```python
from build123d import *

# Parameters (mm, degrees)
CUT_EXTRUDE1_DEPTH      = 20.2
CUT_EXTRUDE1_DEPTH_BACK = 20.2
SKETCH3_R               = 4.05
CUT_EXTRUDE2_DEPTH      = 8.366667
SKETCH4_R               = 4.05
CUT_EXTRUDE3_DEPTH      = 8.366667


with BuildPart() as part:
    # Sketch1 → Revolve1 (revolve)
    with BuildSketch(Plane.XY):
        with BuildLine():
            Line((-1, 8.366666667), (0, 8.366666667))
            Line((0, 8.366666667), (0, 59.633333333))
            Line((0, 59.633333333), (-1, 59.633333333))
            Line((-1, 59.633333333), (-1, 67))
            ThreePointArc((-1, 67), (-1.292893219, 67.707106781), (-2, 68))
            Line((-2, 68), (-5.3, 68))
            Line((-5.3, 68), (-5.3, 57.633333333))
            ThreePointArc((-5.3, 57.633333333), (-4.557500751, 56.319940208), (-4.3, 54.833333333))
            Line((-4.3, 54.833333333), (-4.3, 51.833333333))
            Line((-4.3, 51.833333333), (-6, 51.833333333))
            Line((-6, 51.833333333), (-6, 46.833333333))
            Line((-6, 46.833333333), (-3, 46.833333333))
            Line((-3, 46.833333333), (-3, 44.333333333))
            Line((-3, 44.333333333), (-19.2, 44.333333333))
            Line((-19.2, 44.333333333), (-19.2, 41.333333333))
            Line((-19.2, 41.333333333), (-15.5, 41.333333333))
            Line((-15.5, 41.333333333), (-15.5, 23.666666667))
            Line((-15.5, 23.666666667), (-3, 23.666666667))
            Line((-3, 23.666666667), (-3, 21.166666667))
            Line((-3, 21.166666667), (-6, 21.166666667))
            Line((-6, 21.166666667), (-6, 16.166666667))
            Line((-6, 16.166666667), (-4.3, 16.166666667))
            Line((-4.3, 16.166666667), (-4.3, 13.166666667))
            ThreePointArc((-4.3, 13.166666667), (-4.557500751, 11.680059792), (-5.3, 10.366666667))
            Line((-5.3, 10.366666667), (-5.3, 0))
            Line((-5.3, 0), (-2, 0))
            ThreePointArc((-2, 0), (-1.292893219, 0.292893219), (-1, 1))
            Line((-1, 1), (-1, 8.366666667))
        make_face()
    revolve(axis=Axis((0, 0, 0), (0, 1, 0)))

    # Sketch2 → Cut-Extrude1 (cut, two sides)
    with BuildSketch(Plane.XY) as cut_extrude1_sk:
        with BuildLine():
            Line((1, 8.366666667), (0, 8.366666667))
            Line((0, 8.366666667), (0, 0))
            Line((0, 0), (2, 0))
            ThreePointArc((2, 0), (1.292893219, 0.292893219), (1, 1))
            Line((1, 1), (1, 8.366666667))
        make_face()
        with BuildLine():
            Line((-1, 8.366666667), (-1, 1))
            ThreePointArc((-1, 1), (-1.292893219, 0.292893219), (-2, 0))
            Line((-2, 0), (0, 0))
            Line((0, 0), (0, 8.366666667))
            Line((0, 8.366666667), (-1, 8.366666667))
        make_face()
        with BuildLine():
            Line((-1, 67), (-1, 59.633333333))
            Line((-1, 59.633333333), (1, 59.633333333))
            Line((1, 59.633333333), (1, 67))
            ThreePointArc((1, 67), (1.292893219, 67.707106781), (2, 68))
            Line((2, 68), (-2, 68))
            ThreePointArc((-2, 68), (-1.292893219, 67.707106781), (-1, 67))
        make_face()
    extrude(amount=CUT_EXTRUDE1_DEPTH, mode=Mode.SUBTRACT)
    extrude(cut_extrude1_sk.sketch, amount=-CUT_EXTRUDE1_DEPTH_BACK, mode=Mode.SUBTRACT)

    # Sketch3 → Cut-Extrude2 (cut)
    with BuildSketch(Plane(origin=(0, 68, 0), x_dir=(1, 0, 0), z_dir=(0, 1, 0))):
        Circle(SKETCH3_R)
    extrude(amount=-CUT_EXTRUDE2_DEPTH, mode=Mode.SUBTRACT)

    # Sketch4 → Cut-Extrude3 (cut)
    with BuildSketch(Plane.XZ):
        Circle(SKETCH4_R)
    extrude(amount=-CUT_EXTRUDE3_DEPTH, mode=Mode.SUBTRACT)


solid = part.part
```
CAD build for the part. Positions are in the model's coordinates, mm. A direction names the side the tool comes from. Coordinates: 2 decimals unless noted, no trailing zeros. Order: outer loops, then holes, each group sorted by start corner. A loop starts at its lowest first (then second) coordinate and runs counter-clockwise, first axis right, second up. Notation, with made-up numbers: (-36.5, 2.25) - (-10.5, 2.25) arc R32 ccw to (-10.5, 31.25) - close; hole circle Ø3 at (14.25, -14.5). An arc over 180 degrees is marked (long way). Use a Markdown table: item, result. Add a question column.
(1) Saw through at B-B (z = -12.5). Give the cut face in (x, y).
(2) Which spindle directions (+Z, -Z, +X, -X, +Y, -Y) get a long thin tool onto all of the face, cutting with end or side? Do faces 1 (the face through (13, 41.333, 9)), 2 (the face through (3, 22, 0)), 3 (the face through (-2.45, 62.74, -4.7)), 4 (the face through (4.4, 68, 0.1)). Say none if no direction does.
(3) Saw through at A-A (x = -7). Give the cut face in (y, z).
(4) Saw through at C-C (y = 49). Give the cut face in (x, z), then the cut area to 3 significant figures.
(5) Flat gauge pins, fed straight in: pin 1 (5 mm diameter, centred on y = 19, z = 14.5, fed in from +X); pin 2 (13 mm diameter, centred on x = -2, z = -2.5, fed in from +Y); pin 3 (1 mm diameter, centred on y = 63, z = -4.5, fed in from -X); pin 4 (6 mm diameter, centred on x = -3.5, z = 11, fed in from -Y). Where does each tip first touch, or does it go through?
(6) Drill centre lines: line 1 along X through (y, z) = (61, 2); line 2 along Y through (x, z) = (-3, 4); line 3 along Y through (x, z) = (-7, -3.5). Where is each one in solid material? Low to high. Write a range as [from, to].
(7) Pull direction Z, two halves, no side cores. Call faces 5 (the face through (-4.05, 4.12, 0.07)), 6 (the face through (3, 46, 0)), 7 (the face through (-3, 21.167, -1)): +Z half, -Z half, draft (parallel to the pull), parting line (faces both ways), or undercut.
Solved:
| question | item | result |
|---|---|---|
| 1 | outline | (-14.57, 41.33) - (-9.17, 41.33) - (-9.17, 23.67) - (9.17, 23.67) - (9.17, 41.33) - (14.57, 41.33) - (14.57, 44.33) - (-14.57, 44.33) - close |
| 2 | face 1 | -Y |
| 2 | face 2 | none |
| 2 | face 3 | +Y |
| 2 | face 4 | +Z, -Z, +X, -X, +Y |
| 3 | outline | (23.67, -13.83) - (41.33, -13.83) - (41.33, -17.88) - (44.33, -17.88) - (44.33, 17.88) - (41.33, 17.88) - (41.33, 13.83) - (23.67, 13.83) - close |
| 4 | outline | circle Ø12 at (0, 0) |
| 4 | area | 113 mm² |
| 5 | pin 1 | passes through |
| 5 | pin 2 | stops at y = 68 |
| 5 | pin 3 | stops at x = -3.48 |
| 5 | pin 4 | stops at y = 23.67 |
| 6 | line 1 | x = [-4.91, -3.52], [3.52, 4.91] |
| 6 | line 2 | y = [0, 10.78], [16.17, 21.17], [23.67, 44.33], [46.83, 51.83], [57.22, 68] |
| 6 | line 3 | y = [23.67, 44.33] |
| 7 | face 5 | undercut |
| 7 | face 6 | parting line |
| 7 | face 7 | draft |
